Check sheet for the drawn part. Datum: minimum x, y, z corner. Units: mm. A direction names the side the tool comes from. Give positions to 0.01 mm unless a question says otherwise; leave off trailing zeros. Write each loop counter-clockwise with the first axis right and the second up, starting at its lowest first coordinate (ties: lowest second). Pieces come first, ordered by that corner, then holes. Notation, with made-up numbers: M 38,-17 L 97,-17 A31 cw 97,17 Z; hole C -26,55 d11. An arc over 180 degrees is marked long. Use CSV: the item, a comma, the result in double quotes. Start each with the question number.
1. Cross-section at C-C, the plane x = 16. Enter the section's corners in (y, z), and give its area (3 significant figures).
2. Depth check by flat-ended pin: P1, Ø10, axis at x = 34.5, z = 13.5, coming from the +Y side; P2, Ø8, axis at x = 19, z = 30, coming from the -Y side; P3, Ø3, axis at y = 37.5, z = 26, coming from the +X side. Enter the tip coordinate at first touch or a pass-through.
3. Cross-section at D-D, the plane y = 44.5. Enter the section's corners in (x, z).
4. Cross-section at B-B, the plane y = 15. Enter the section's corners in (x, z), and give its area (3 significant figures).
5. Scan lines: line 1 (X direction, y = 28.5, z = 20); line 2 (X direction, y = 19.75, z = 20); line 3 (Z direction, x = 20, y = 15.5). Record each from-to range of solid material in increasing order.
6. Access from +Z, -Z, +X, -X, +Y, -Y to the whole of each face (thin tool, end or side, straight path). Record for the marked faces 1, 2 and 3.
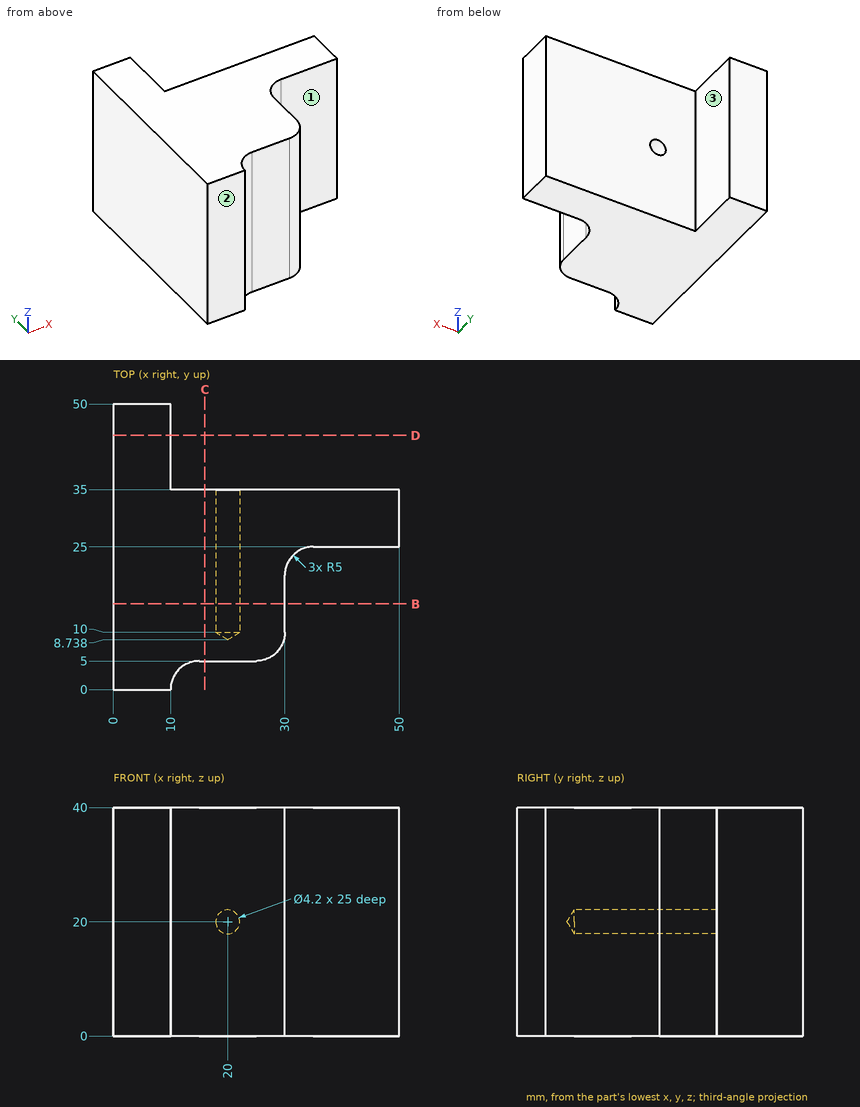
Worked answers:
1,outline,"M 5,0 L 35,0 L 35,40 L 5,40 Z"
1,area,"1,200 mm^2"
2,P1,"stops at y = 35"
2,P2,"stops at y = 5"
2,P3,"stops at x = 10"
3,outline,"M 0,0 L 10,0 L 10,40 L 0,40 Z"
4,outline,"M 0,0 L 30,0 L 30,40 L 0,40 Z; hole C 20,20 d4.2"
4,area,"1,190 mm^2"
5,line 1,"x = 0 to 17.9, 22.1 to 50"
5,line 2,"x = 0 to 17.9, 22.1 to 30"
5,line 3,"z = 0 to 17.9, 22.1 to 40"
6,face 1,"+Z, -Z, +X, -Y"
6,face 2,"+Z, -Z, +X, -X, -Y"
6,face 3,"+Z, -Z, +X, +Y"
